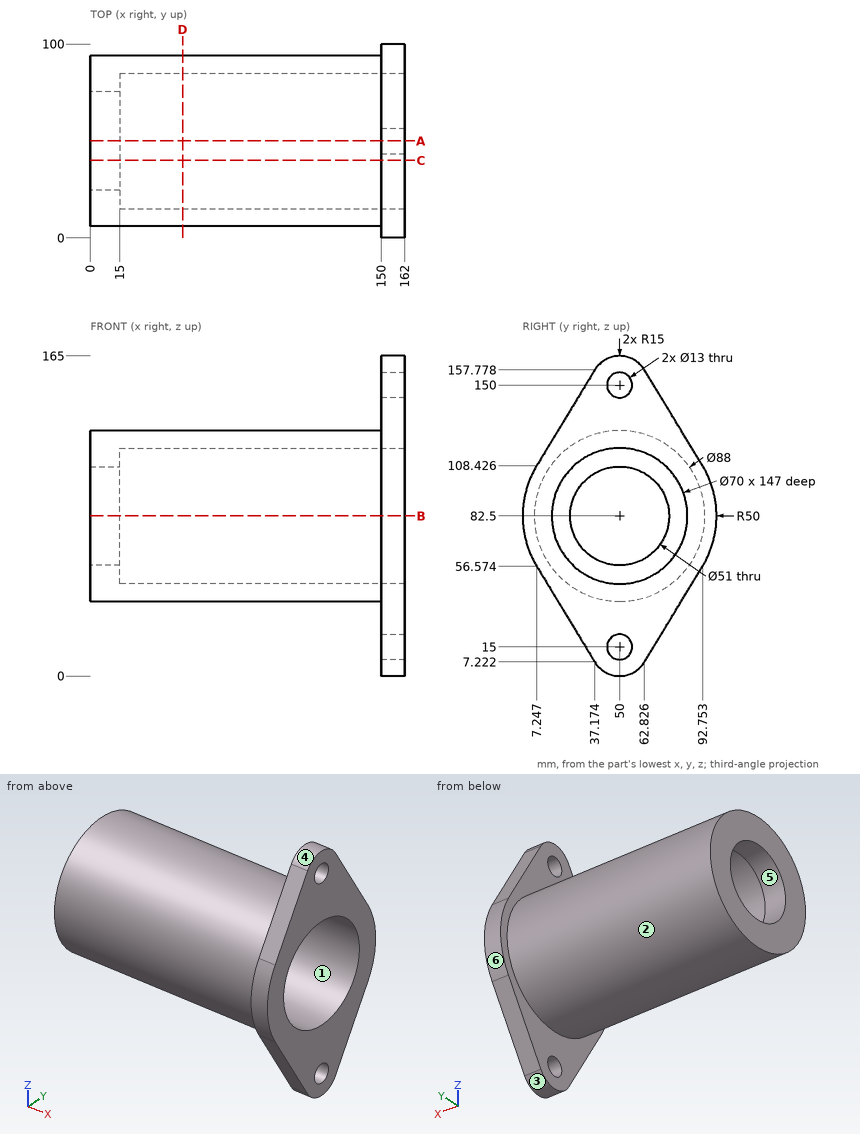
Input: dimensioned drawing with shaded views. Units: mm. Origin: part minimum x, y, z. A direction names the side the tool comes from. Round coordinates to 2 decimals unless told otherwise and drop trailing zeros. Loops run counter-clockwise (first coordinate to the right, second up) from the corner with the lowest first, then second, coordinate; pieces in that order, holes last. Notation, with made-up numbers: (89, 0) -> (123, 0) arc R30 cw to (123, 30) -> close; hole circle Ø3 at (-22, -31.5). An arc over 180 degrees is marked (long way). Answer as a JSON object with one key per item and string values. Group by question number.
1) Ray query, L1, parallel to Y at x = 57.5, z = 82.5; L2, parallel to X at y = 26.5, z = 69.5; L3, parallel to Y at x = 46.5, z = 67. Return the intervals inside material, ascending.
2) Section query B-B on z = 82.5. Output: boundary loops of the cut face in (x, y), plus the area to 4 significant figures.
3) Draft query along Y for the marked faces 4, 5 and 6. Return one class per face: +Y half, -Y half, draft (parallel to the pull), parting line (faces both ways), or undercut.
4) Section query A-A on y = 50. Output: boundary loops of the cut face in (x, z), plus the area to 3 significant figures.
5) Pin query (flat end, axial travel): pin 1 (3 mm diameter, centred on x = 138.5, y = 44, fed in from +Z); pin 2 (3 mm diameter, centred on x = 114.5, y = 15, fed in from -Z) (1 decimal); pin 3 (4 mm diameter, centred on x = 49.5, y = 49.5, fed in from +Z). Return the tip coordinate at first contact, or that it passes through.
6) Section query C-C on y = 40. Output: boundary loops of the cut face in (x, z), plus the area to 3 significant figures.
7) Reachability of the marked faces 1, 2 and 3 from +Z, -Z, +X, -X, +Y, -Y: full face, straight path, thin tool, end or side. Return the list, or none.
8) Section query D-D on x = 47.5. Output: boundary loops of the cut face in (y, z).
Reply:
{
 "1": {"L1": "y = 6 to 15, 85 to 94", "L2": "x = 0 to 15", "L3": "y = 8.82 to 18.62, 81.38 to 91.18"},
 "2": {"outline": "(0, 6) -> (150, 6) -> (150, 0) -> (162, 0) -> (162, 15) -> (15, 15) -> (15, 24.5) -> (0, 24.5) -> close; (0, 75.5) -> (15, 75.5) -> (15, 85) -> (162, 85) -> (162, 100) -> (150, 100) -> (150, 94) -> (0, 94) -> close", "area": "3,345 mm2"},
 "3": {"face 4": "parting line", "face 5": "undercut", "face 6": "+Y half"},
 "4": {"outline": "(0, 38.5) -> (150, 38.5) -> (150, 21.5) -> (162, 21.5) -> (162, 47.5) -> (15, 47.5) -> (15, 57) -> (0, 57) -> close; (0, 108) -> (15, 108) -> (15, 117.5) -> (162, 117.5) -> (162, 143.5) -> (150, 143.5) -> (150, 126.5) -> (0, 126.5) -> close; (150, 0) -> (162, 0) -> (162, 8.5) -> (150, 8.5) -> close; (150, 156.5) -> (162, 156.5) -> (162, 165) -> (150, 165) -> close", "area": "3,810 mm2"},
 "5": {"pin 1": "stops at z = 126.27", "pin 2": "stops at z = 54", "pin 3": "stops at z = 126.5"},
 "6": {"outline": "(0, 39.65) -> (150, 39.65) -> (150, 3.82) -> (162, 3.82) -> (162, 48.96) -> (15, 48.96) -> (15, 59.04) -> (0, 59.04) -> close; (0, 105.96) -> (15, 105.96) -> (15, 116.04) -> (162, 116.04) -> (162, 161.18) -> (150, 161.18) -> (150, 125.35) -> (0, 125.35) -> close", "area": "4,180 mm2"},
 "7": {"face 1": "+X", "face 2": "-X", "face 3": "-Z, +X, -X"},
 "8": {"outline": "circle Ø88 at (50, 82.5); hole circle Ø70 at (50, 82.5)"}
}
